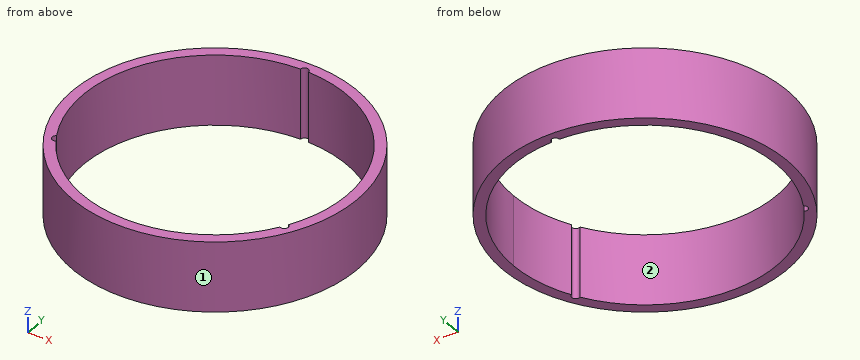
from build123d import *

# Parameters (mm, degrees)
SKETCH1_R           = 81
BOSS_EXTRUDE1_DEPTH = 40


with BuildPart() as part:
    # Sketch1 → Boss-Extrude1 (new body)
    with BuildSketch(Plane.XY):
        Circle(SKETCH1_R)
        with BuildLine():
            ThreePointArc((2.231689825, 74.966789717), (53.816246324, 52.238028596), (75, 0))
            ThreePointArc((75, 0), (72.725250751, -18.331336645), (66.038989248, -35.550694777))
            ThreePointArc((66.038989248, -35.550694777), (66.876463055, -36.369681556), (67.1838422, -37.5))
            ThreePointArc((67.1838422, -37.5), (66.053461983, -39.441163372), (63.807299423, -39.416094941))
            ThreePointArc((63.807299423, -39.416094941), (0, -75), (-63.807299423, -39.416094941))
            ThreePointArc((-63.807299423, -39.416094941), (-66.884819353, -38.615968458), (-66.038989248, -35.550694777))
            ThreePointArc((-66.038989248, -35.550694777), (-64.951905284, 37.5), (-2.231689825, 74.966789717))
            ThreePointArc((-2.231689825, 74.966789717), (-0.016605601, 77.231875143), (2.231936916, 75))
            ThreePointArc((2.231936916, 75), (2.231875143, 74.983394399), (2.231689825, 74.966789717))
        make_face(mode=Mode.SUBTRACT)
    extrude(amount=BOSS_EXTRUDE1_DEPTH)


solid = part.part
Work out the finished part from the listing and answer in its coordinate system (mm). Face numbers are marked on the shaded views. Give positions to 0.01 mm unless a question says otherwise; leave off trailing zeros. Loops run counter-clockwise (first coordinate to the right, second up) from the corner with the lowest first, then second, coordinate; pieces in that order, holes last. Notation, with made-up numbers: M -19,59 L 30,59 A14 cw 30,82 Z; hole C 75,70.5 d8. An arc over 180 degrees is marked long. Use CSV: the item, a comma, the result in double quotes.
1) Determine the mould class of the marked faces 1 and 2 for opening direction X: released by +X, released by -X, zero draft, split by the parting line, or undercut.
Answer:
face 1,"split by the parting line"
face 2,"undercut"
2) Given P1, Ø1.5, axis at y = -54.5, z = 6.5, coming from the +X side; P2, Ø1.5, axis at y = 61.5, z = 25, coming from the -X side; P3, Ø2, axis at x = 63, z = 32, coming from the +Y side, each flat-ended and moving along its own axis, determine where each tip first touches the part or whether it passes through.
Answer:
P1,"x = 60.6"
P2,"x = -53.58"
P3,"y = 52.12"
3) Find section B-B on y = 40.5. Write down the section's boundary in (x, z).
Answer:
outline,"M -70.15,0 L -63.12,0 L -63.12,40 L -70.15,40 Z; M 63.12,0 L 70.15,0 L 70.15,40 L 63.12,40 Z"
4) Consider L1, parallel to Y at x = -29.5, z = 17; L2, parallel to Y at x = -56.5, z = 6; L3, parallel to X at y = -17.5, z = 14.5. Determine where each line is inside the solid, lowest interval first.
Answer:
L1,"-75.44 to -68.95, 68.95 to 75.44"
L2,"-58.04 to -49.32, 49.32 to 58.04"
L3,"-79.09 to -72.93, 72.93 to 79.09"
5) Find section A-A on x = 0. Write down the section's boundary in (y, z).
Answer:
outline,"M -81,0 L -75,0 L -75,40 L -81,40 Z; M 77.23,0 L 81,0 L 81,40 L 77.23,40 Z"
